Work out the finished part from the listing and answer in its coordinate system (mm). A direction names the side the tool comes from. Coordinates: 2 decimals unless noted, no trailing zeros. Order: outer loops, then holes, each group sorted by start corner. A loop starts at its lowest first (then second) coordinate and runs counter-clockwise, first axis right, second up. Notation, with made-up numbers: (61, 39) - (75, 39) arc R26 cw to (75, 57) - close; hole circle Ø6 at (84.5, 28). An arc over 180 degrees is marked (long way). Answer as a JSON object with one key per item and string values. Group by question number.
1) Find the intervals of material crossed by line 1 along Y through (x, z) = (2.5, -11.25); line 2 along X through (y, z) = (5, -8); line 3 along Z through (x, y) = (7.75, 4), in increasing order.
2) Section D-D (x = 3.25) is taken. Give the vertices of the cut face in (y, z), plus the area to 3 significant figures.
3) Section A-A (z = -6) is taken. Give the vertices of the cut face in (x, y) (3 decimals), plus the area to 3 significant figures.
4) Section C-C (y = 3.75) is taken. Give the vertices of the cut face in (x, z) (3 decimals).
5) A tool of negligible diameter and unlimited length cuts with its end or side. For faces 1 (the face through (5.49, 4.48, -3.68)), 2 (the face through (11.1, 1.39, -0.86)), from which of +Z, -Z, +X, -X, +Y, -Y can it reach the whole face along a straight path? Write none if from no direction.
6) Each of these flat-tipped pins is pushed along its axis until it touches: P1, Ø3, axis at x = 4, y = 5, coming from the +Z side; P2, Ø1.5, axis at y = 3, z = -10.5, coming from the +X side. Where does it stop, or does it pass through?
7) Section B-B (x = 6) is taken. Give the vertices of the cut face in (y, z) (3 decimals), plus the area to 3 significant figures.
from build123d import *

# Parameters (mm, degrees)
SKETCH1_W           = 12
SKETCH1_H           = 12
BOSS_EXTRUDE1_DEPTH = 2.75
SKETCH3_R           = 2.375
BOSS_EXTRUDE2_DEPTH = 3.5
FILLET1_R           = 3


with BuildPart() as part:
    # Sketch1 → Boss-Extrude1 (new body)
    with BuildSketch(Plane(origin=(0, 0, 0), x_dir=(1, 0, 0), z_dir=(0, 1, 0))):
        with Locations((6, 6)):
            Rectangle(SKETCH1_W, SKETCH1_H)
    extrude(amount=BOSS_EXTRUDE1_DEPTH)

    # Sketch3 → Boss-Extrude2 (add)
    with BuildSketch(Plane(origin=(0, 2.75, 0), x_dir=(1, 0, 0), z_dir=(0, 1, 0))):
        with Locations((6, 6)):
            Circle(SKETCH3_R)
    extrude(amount=BOSS_EXTRUDE2_DEPTH)

    # Fillet1
    fillet1_edges = [part.edges().sort_by_distance(p)[0] for p in [
        (0, 1.375, -12),
        (12, 1.375, -12),
        (12, 1.375, 0),
        (0, 1.375, 0),
    ]]
    fillet(fillet1_edges, radius=FILLET1_R)


solid = part.part
Report:
{
 "1": {"line 1": "y = 0 to 2.75", "line 2": "x = 4.72 to 7.28", "line 3": "z = -7.61 to -4.39"},
 "2": {"outline": "(0, -12) - (2.75, -12) - (2.75, 0) - (0, 0) - close", "area": "33.0 mm²"},
 "3": {"outline": "(0, 0) - (12, 0) - (12, 2.75) - (8.375, 2.75) - (8.375, 6.25) - (3.625, 6.25) - (3.625, 2.75) - (0, 2.75) - close", "area": "49.6 mm²"},
 "4": {"outline": "circle Ø4.75 at (6, -6)"},
 "5": {"face 1": "+Y", "face 2": "+Z, +X, +Y, -Y"},
 "6": {"P1": "stops at z = -3.68", "P2": "stops at x = 11.89"},
 "7": {"outline": "(0, -12) - (2.75, -12) - (2.75, -8.375) - (6.25, -8.375) - (6.25, -3.625) - (2.75, -3.625) - (2.75, 0) - (0, 0) - close", "area": "49.6 mm²"}
}
